Geometry check sheet. Reference: the model listing, model coordinates, mm. Coordinates: 2 decimals unless noted, no trailing zeros. Write each loop counter-clockwise with the first axis right and the second up, starting at its lowest first coordinate (ties: lowest second). Pieces come first, ordered by that corner, then holes.
from build123d import *

# Parameters (mm, degrees)
F0_W        = 127
F0_H        = 152.4
F0_R        = 4.25
F1_DEPTH    = 38.1
F3_R        = 3.96875
F4_DEPTH    = 50.8
F5_R        = 6.25
F5_R_2      = 4.25
F5_R_3      = 5.96875
F5_R_4      = 3.96875
F6_DEPTH    = 12.7
F7_C1_SIZE  = 2.54
F7_C2_SIZE  = 2.54
F7_C3_SIZE  = 2.54
F7_C4_SIZE  = 2.54
F7_C5_SIZE  = 2.54
F7_C6_SIZE  = 2.54
F7_C7_SIZE  = 2.54
F7_C8_SIZE  = 2.54
F7_C9_SIZE  = 2.54
F7_C10_SIZE = 2.54
F7_C11_SIZE = 2.54
F7_C12_SIZE = 2.54
F7_C13_SIZE = 2.54
F7_C14_SIZE = 2.54
F7_C15_SIZE = 2.54
F7_C16_SIZE = 2.54


# Not quite as in the source:
# - two fillets or chamfers of one size are made in one step
# - a feature names something its author has since deleted; it is built from what else it names


with BuildPart() as f1:
    # F0 (on Top) → F1 (new body)
    with BuildSketch(Plane.XY):
        Rectangle(F0_W, F0_H)
        Circle(F0_R, mode=Mode.SUBTRACT)
    extrude(amount=F1_DEPTH)

    # F3 (on face) → F4 (cut)
    with BuildSketch(Plane.XY.offset(38.1)):
        with Locations((0, -63.5)):
            Circle(F3_R)
    extrude(amount=-F4_DEPTH, mode=Mode.SUBTRACT)

    # F5 (on face) → F6 (cut)
    with BuildSketch(Plane(origin=(0, 0, 0), x_dir=(1, 0, 0), z_dir=(0, 0, -1))):
        Circle(F5_R)
        Circle(F5_R_2, mode=Mode.SUBTRACT)
        with Locations((0, 63.5)):
            Circle(F5_R_3)
        with Locations((0, 63.5)):
            Circle(F5_R_4, mode=Mode.SUBTRACT)
    extrude(amount=-F6_DEPTH, mode=Mode.SUBTRACT)

    # F7: chamfer of 2.54 on 16 edges, made by hand

    # F7_c1
    f7_c1_edges = [f1.edges().sort_by_distance(p)[0] for p in [
        (-63.5, -76.2, 19.05),
    ]]
    chamfer(f7_c1_edges, length=F7_C1_SIZE)

    # F7_c2
    f7_c2_edges = [f1.edges().sort_by_distance(p)[0] for p in [
        (63.5, -76.2, 19.05),
    ]]
    chamfer(f7_c2_edges, length=F7_C2_SIZE)

    # F7_c3
    f7_c3_edges = [f1.edges().sort_by_distance(p)[0] for p in [
        (0, -76.2, 0),
    ]]
    chamfer(f7_c3_edges, length=F7_C3_SIZE)

    # F7_c4
    f7_c4_edges = [f1.edges().sort_by_distance(p)[0] for p in [
        (0, -76.2, 38.1),
    ]]
    chamfer(f7_c4_edges, length=F7_C4_SIZE)

    # F7_c5
    f7_c5_edges = [f1.edges().sort_by_distance(p)[0] for p in [
        (-63.5, 76.2, 19.05),
    ]]
    chamfer(f7_c5_edges, length=F7_C5_SIZE)

    # F7_c6
    f7_c6_edges = [f1.edges().sort_by_distance(p)[0] for p in [
        (-63.5, 0, 0),
    ]]
    chamfer(f7_c6_edges, length=F7_C6_SIZE)

    # F7_c7
    f7_c7_edges = [f1.edges().sort_by_distance(p)[0] for p in [
        (-63.5, 0, 38.1),
    ]]
    chamfer(f7_c7_edges, length=F7_C7_SIZE)

    # F7_c8
    f7_c8_edges = [f1.edges().sort_by_distance(p)[0] for p in [
        (63.5, 76.2, 19.05),
    ]]
    chamfer(f7_c8_edges, length=F7_C8_SIZE)

    # F7_c9
    f7_c9_edges = [f1.edges().sort_by_distance(p)[0] for p in [
        (63.5, 0, 0),
    ]]
    chamfer(f7_c9_edges, length=F7_C9_SIZE)

    # F7_c10
    f7_c10_edges = [f1.edges().sort_by_distance(p)[0] for p in [
        (63.5, 0, 38.1),
    ]]
    chamfer(f7_c10_edges, length=F7_C10_SIZE)

    # F7_c11
    f7_c11_edges = [f1.edges().sort_by_distance(p)[0] for p in [
        (0, 76.2, 0),
    ]]
    chamfer(f7_c11_edges, length=F7_C11_SIZE)

    # F7_c12
    f7_c12_edges = [f1.edges().sort_by_distance(p)[0] for p in [
        (-5.96875, -63.5, 0),
    ]]
    chamfer(f7_c12_edges, length=F7_C12_SIZE)

    # F7_c13
    f7_c13_edges = [f1.edges().sort_by_distance(p)[0] for p in [
        (-6.25, 0, 0),
    ]]
    chamfer(f7_c13_edges, length=F7_C13_SIZE)

    # F7_c14
    f7_c14_edges = [f1.edges().sort_by_distance(p)[0] for p in [
        (0, 76.2, 38.1),
    ]]
    chamfer(f7_c14_edges, length=F7_C14_SIZE)

    # F7_c15
    f7_c15_edges = [f1.edges().sort_by_distance(p)[0] for p in [
        (-3.96875, -63.5, 38.1),
    ]]
    chamfer(f7_c15_edges, length=F7_C15_SIZE)

    # F7_c16
    f7_c16_edges = [f1.edges().sort_by_distance(p)[0] for p in [
        (-4.25, 0, 38.1),
    ]]
    chamfer(f7_c16_edges, length=F7_C16_SIZE)


solid = f1.part
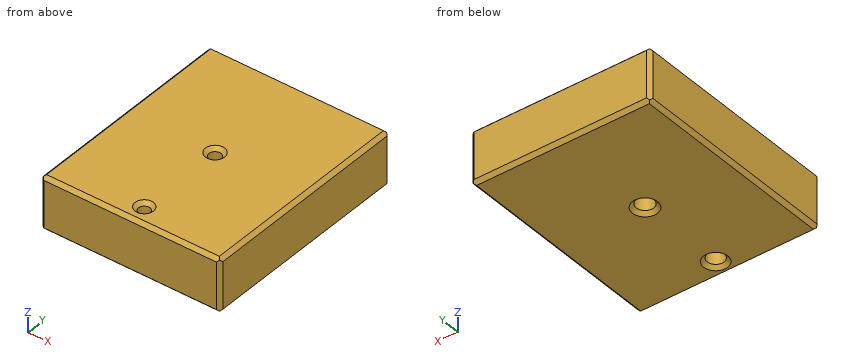
1. Sectioned sample at C-C, the plane y = -63.5. Record the boundary of the cut face in (x, z), and give its area (3 significant figures).
Computed values:
outline: (-63.5, 2.54) - (-60.96, 0) - (-8.51, 0) - (-5.97, 2.54) - (-5.97, 12.7) - (-3.97, 12.7) - (-3.97, 35.56) - (-6.51, 38.1) - (-60.96, 38.1) - (-63.5, 35.56) - close; (3.97, 12.7) - (5.97, 12.7) - (5.97, 2.54) - (8.51, 0) - (60.96, 0) - (63.5, 2.54) - (63.5, 35.56) - (60.96, 38.1) - (6.51, 38.1) - (3.97, 35.56) - close
area: 4,460 mm2
2. Thickness scan on line 1 along Y through (x, z) = (0, 27.5); line 2 along X through (y, z) = (0, 22); line 3 along Y through (x, z) = (0, 7.25). Record the ranges inside material, lowest first.
Computed values:
line 1: y = -76.2 to -67.47, -59.53 to -4.25, 4.25 to 76.2
line 2: x = -63.5 to -4.25, 4.25 to 63.5
line 3: y = -76.2 to -69.47, -57.53 to -6.25, 6.25 to 76.2
3. Sectioned sample at A-A, the plane y = 0. Record the boundary of the cut face in (x, z).
Computed values:
outline: (-63.5, 2.54) - (-60.96, 0) - (-8.79, 0) - (-6.25, 2.54) - (-6.25, 12.7) - (-4.25, 12.7) - (-4.25, 35.56) - (-6.79, 38.1) - (-60.96, 38.1) - (-63.5, 35.56) - close; (4.25, 12.7) - (6.25, 12.7) - (6.25, 2.54) - (8.79, 0) - (60.96, 0) - (63.5, 2.54) - (63.5, 35.56) - (60.96, 38.1) - (6.79, 38.1) - (4.25, 35.56) - close
4. Gauge pin test, flat ends, axial feed: pin 1 Ø4 at (x, y) = (-1, -2.5) entering from -Z; pin 2 Ø9.5 at (x, y) = (0, -62) entering from -Z. Record the tip position at first contact, or that the pin passes through.
Computed values:
pin 1: stops at z = 12.7
pin 2: stops at z = 2.26
5. Sectioned sample at B-B, the plane x = 0. Give the number of separate pieces and of enclosed holes in the cut face, and give its area (3 significant figures).
Computed values:
separate pieces: 3
enclosed holes: 0
area: 5,040 mm2
